Autodesk Inventor part; units mm, degrees
ref_plane "YZ Plane" through (0, 0, 0) normal (1, 0, 0) x (0, 1, 0)
ref_plane "XZ Plane" through (0, 0, 0) normal (0, 1, 0) x (-1, 0, 0)
ref_plane "XY Plane" through (0, 0, 0) normal (0, 0, 1) x (1, 0, 0)
sketch "Sketch1" plane through (0, 0, 0) normal (0, 0, 1) x (1, 0, 0)
  line L0 (0, 0) -> (306.07, 0)
  line L1 (306.07, 0) -> (306.07, 208.28)
  line L2 (306.07, 208.28) -> (0, 208.28)
  line L3 (0, 208.28) -> (0, 0)
  dimension "d0" = 306.07
  dimension "d1" = 208.28
extrude "Extrusion1" add sketch "Sketch1" along normal blind 12.7
sketch "Sketch2" plane through (0, 0, 12.7) normal (0, 0, 1) x (1, 0, 0)
  circle A0 centre (38.1, 31.75) radius 4.1656
  circle A1 centre (267.97, 31.75) radius 4.1656
  line L0 (306.07, 0) -> (306.07, 208.28)
  line L1 (0, 208.28) -> (0, 0)
  line L2 (0, 0) -> (306.07, 0)
  dimension "d4" = 8.3312
  dimension "d5" = 8.3312
  dimension "d6" = 38.1
  dimension "d7" = 38.1
  dimension "d8" = 31.75
  dimension "d9" = 31.75
extrude "Extrusion2" cut sketch "Sketch2" against normal blind 25.4
properties part number "rear angled wall"
Could you check a few things on this model? Use its own coordinates, in mm. Round coordinates to 2 decimals unless told otherwise and drop trailing zeros. Write each loop counter-clockwise with the first axis right and the second up, starting at its lowest first coordinate (ties: lowest second). Pieces come first, ordered by that corner, then holes. Notation, with made-up numbers: (-5.5, -34.5) - (4.5, -34.5) arc R22 cw to (4.5, -0.5) - close; hole circle Ø9 at (49, 58.25). An arc over 180 degrees is marked (long way). Use a Markdown table: item, result.
Q1. I want a section at B-B (x = 38.1). List the corners of the cut face in (y, z) for me.
Output values:
| item | result |
|---|---|
| outline | (0, 0) - (27.58, 0) - (27.58, 12.7) - (0, 12.7) - close; (35.92, 0) - (208.28, 0) - (208.28, 12.7) - (35.92, 12.7) - close |
Q2. Please list where this line runs through material, in increasing order: L1, parallel to Y at x = 267.97, z = 6.
Output values:
| item | result |
|---|---|
| L1 | 0 to 27.58, 35.92 to 208.28 |
Q3. Thinking about a two-plate mould opening in Y: for faces 1 (the cylindrical face through (33.94, 31.93, 6.44)), 2 (the flat face through (151, 0, 6)), 3 (the flat face through (151, 106, 0)), which applies, released by +Y, released by -Y, zero draft, split by the parting line, or undercut?
Output values:
| item | result |
|---|---|
| face 1 | undercut |
| face 2 | released by -Y |
| face 3 | zero draft |
Q4. I want a section at A-A (y = 31.75). List the corners of the cut face in (x, z) for me, plus the area to 3 significant figures.
Output values:
| item | result |
|---|---|
| outline | (0, 0) - (33.93, 0) - (33.93, 12.7) - (0, 12.7) - close; (42.27, 0) - (263.8, 0) - (263.8, 12.7) - (42.27, 12.7) - close; (272.14, 0) - (306.07, 0) - (306.07, 12.7) - (272.14, 12.7) - close |
| area | 3,680 mm2 |
Q5. For pin 1 (4 mm diameter, centred on y = 135.5, z = 11.5, fed in from -X), with a flat end and sliding along its axis, tell me the tip position at first contact or that it passes through.
Output values:
| item | result |
|---|---|
| pin 1 | x = 0 |
